Here's how the part is built. I have some questions about the finished solid (model axes, mm). A direction names the side the tool comes from. Round coordinates to 2 decimals unless told otherwise and drop trailing zeros. Order: outer loops, then holes, each group sorted by start corner. A loop starts at its lowest first (then second) coordinate and runs counter-clockwise, first axis right, second up. Notation, with made-up numbers: (-22.75, -25) -> (27.25, -25) arc R36 cw to (27.25, 9) -> close; hole circle Ø7 at (31.25, 87.25). An arc over 180 degrees is marked (long way). Use a Markdown table: item, result. Add a question column.
(1) If I drill on probe 1 along Y at (x, z) = (11, 17.5); probe 2 along Z at (x, y) = (-11, -27) (3 decimals); probe 3 along X at (y, z) = (-34, 2) (3 decimals), over which ranges is the centre line in solid material (lowest first)?
(2) I'm going to push flat-ended pins straight in: P1, Ø11, axis at x = 32, z = 27.5, coming from the -Y side; P2, Ø1.7, axis at x = 58, y = -24.5, coming from the -Z side; P3, Ø0.6, axis at x = 58, y = 24.5, coming from the -Z side. Where does each tip first touch, or does it pass through?
(3) I want a section at A-A, the plane z = 7.5. Please give me the cut outline in (x, y) (3 decimals), then the cut area to 3 significant figures.
(4) On a 3-axis mill with a long thin cutter (end or side, diameter ignored), from which of +Z, -Z, +X, -X, +Y, -Y can I reach the whole of each face in a straight line? I mean faces 1 (the face through (0, 63.5, 0)), 2 (the face through (0, -63.5, 0)), 3 (the face through (32.73, 16.55, 51.97)), 4 (the face through (80, 0, 38.1)), 5 (the face through (22.225, -17, 18)). Say none if no direction works.
(5) I want a section at C-C, the plane x = 75.5. Please give me the cut outline in (y, z) (3 decimals).
(6) I want a section at B-B, the plane y = -43.5. Please give me the cut outline in (x, z) (3 decimals), then the cut area to 3 significant figures.
from build123d import *

# Parameters (mm, degrees)
F1_DEPTH = 63.5
F2_DEPTH = 25.4
F3_DEPTH = 7.9375
F5_R     = 6.35


with BuildPart() as f1:
    # F0 (on Front) → F1 (new body, symmetric)
    with BuildSketch(Plane.XZ):
        Polygon((-41.275, -9.525), (41.275, -9.525), (41.275, 9.525), (22.225, 9.525), (-41.275, 9.525), align=None)
    extrude(amount=F1_DEPTH, both=True)

    # F0 (on Front) → F2 (join, symmetric)
    with BuildSketch(Plane.XZ):
        with BuildLine():
            Line((22.225, 9.525), (41.275, 9.525))
            Line((41.275, 9.525), (41.275, 27.0002))
            ThreePointArc((41.275, 27.0002), (45.92468, 38.22552), (57.15, 42.8752))
            Line((57.15, 42.8752), (60.325, 42.8752))
            Line((60.325, 42.8752), (60.325, 61.9252))
            Line((60.325, 61.9252), (57.15, 61.9252))
            ThreePointArc((57.15, 61.9252), (32.454296, 51.695904), (22.225, 27.0002))
            Line((22.225, 27.0002), (22.225, 9.525))
        make_face()
    extrude(amount=F2_DEPTH, both=True)

    # F0 (on Front) → F3 (join, symmetric)
    with BuildSketch(Plane.XZ):
        with BuildLine():
            add(Edge.make_bspline(
                [(-41.275, 9.525), (-43.483493, 41.179909), (17.105941, 54.288729), (60.325, 66.675)],
                knots=[0, 0, 0, 0, 116.570504, 116.570504, 116.570504, 116.570504], degree=3))
            Line((-41.275, 9.525), (22.225, 9.525))
            Line((22.225, 9.525), (22.225, 27.0002))
            ThreePointArc((22.225, 27.0002), (32.454296, 51.695904), (57.15, 61.9252))
            Line((57.15, 61.9252), (60.325, 61.9252))
            Line((60.325, 61.9252), (60.325, 66.675))
        make_face()
    extrude(amount=F3_DEPTH, both=True)

    # F0 (on Front) → F4 (revolve)
    with BuildSketch(Plane.XZ):
        Polygon((111.125, 66.675), (79.115786, 66.675), (79.115786, 61.9252), (79.115786, 42.8752), (79.115786, 38.1), (111.125, 38.1), align=None)
    revolve(axis=Axis((79.115786, 0, 52.3875), (0, 0, 1)))

    # F5
    f5_edges = [f1.edges().sort_by_distance(p)[0] for p in [
        (41.275, -63.5, 0),
        (-41.275, -63.5, 0),
        (-41.275, 63.5, 0),
        (41.275, 63.5, 0),
    ]]
    fillet(f5_edges, radius=F5_R)


solid = f1.part
Taken from the geometry:
| question | item | result |
|---|---|---|
| 1 | probe 1 | y = -7.94 to 7.94 |
| 1 | probe 2 | z = -9.525 to 9.525 |
| 1 | probe 3 | x = -41.275 to 41.275 |
| 2 | P1 | stops at y = -25.4 |
| 2 | P2 | stops at z = 38.1 |
| 2 | P3 | stops at z = 42.88 |
| 3 | outline | (-41.275, -57.15) arc R6.35 ccw to (-34.925, -63.5) -> (34.925, -63.5) arc R6.35 ccw to (41.275, -57.15) -> (41.275, 57.15) arc R6.35 ccw to (34.925, 63.5) -> (-34.925, 63.5) arc R6.35 ccw to (-41.275, 57.15) -> close |
| 3 | area | 10,400 mm2 |
| 4 | face 1 | +Z, -Z, +X, -X, +Y |
| 4 | face 2 | +Z, -Z, +X, -X, -Y |
| 4 | face 3 | +Z, -X, +Y |
| 4 | face 4 | -Z, +X, +Y, -Y |
| 4 | face 5 | +Z, -X, -Y |
| 5 | outline | (-31.804, 38.1) -> (31.804, 38.1) -> (31.804, 66.675) -> (-31.804, 66.675) -> close |
| 6 | outline | (-41.275, -9.525) -> (41.275, -9.525) -> (41.275, 9.525) -> (-41.275, 9.525) -> close |
| 6 | area | 1,570 mm2 |
